Geometry: final body of the model. Coordinates: model frame, mm. Give positions to 0.01 mm unless a question says otherwise; leave off trailing zeros. Order: outer loops, then holes, each group sorted by start corner. A loop starts at its lowest first (then second) coordinate and runs counter-clockwise, first axis right, second up. Notation, with made-up numbers: (-17, -31) -> (8, -31) arc R20 cw to (8, -8) -> close; hole circle Ø2 at (81.5, 83). An arc over 180 degrees is marked (long way). Write item = value, one per line.
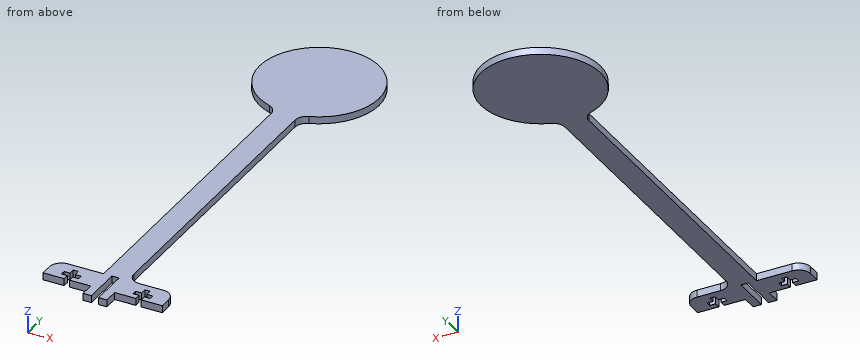
```python
from build123d import *

# Parameters (mm, degrees)
BOSS_EXTRUDE1_DEPTH = 3
FILLET1_R           = 5


with BuildPart() as part:
    # Sketch1 → Boss-Extrude1 (new body)
    with BuildSketch(Plane.XY):
        with BuildLine():
            Line((-5, -25), (-5, -159))
            Line((-5, -159), (-25, -159))
            Line((-25, -159), (-25, -169))
            Line((-25, -169), (-16.1, -169))
            Line((-16.1, -169), (-16.1, -166.5))
            Line((-16.1, -166.5), (-18.6, -166.5))
            Line((-18.6, -166.5), (-18.6, -164.5))
            Line((-18.6, -164.5), (-16.1, -164.5))
            Line((-16.1, -164.5), (-16.1, -162))
            Line((-16.1, -162), (-13.9, -162))
            Line((-13.9, -162), (-13.9, -164.5))
            Line((-13.9, -164.5), (-11.4, -164.5))
            Line((-11.4, -164.5), (-11.4, -166.5))
            Line((-11.4, -166.5), (-13.9, -166.5))
            Line((-13.9, -166.5), (-13.9, -169))
            Line((-13.9, -169), (-5, -169))
            Line((-5, -169), (-5, -175))
            Line((-5, -175), (-1.5, -175))
            Line((-1.5, -175), (-1.5, -159))
            Line((-1.5, -159), (1.5, -159))
            Line((1.5, -159), (1.5, -175))
            Line((1.5, -175), (5, -175))
            Line((5, -175), (5, -169))
            Line((5, -169), (13.9, -169))
            Line((13.9, -169), (13.9, -166.5))
            Line((13.9, -166.5), (11.4, -166.5))
            Line((11.4, -166.5), (11.4, -164.5))
            Line((11.4, -164.5), (13.9, -164.5))
            Line((13.9, -164.5), (13.9, -162))
            Line((13.9, -162), (16.1, -162))
            Line((16.1, -162), (16.1, -164.5))
            Line((16.1, -164.5), (18.6, -164.5))
            Line((18.6, -164.5), (18.6, -166.5))
            Line((18.6, -166.5), (16.1, -166.5))
            Line((16.1, -166.5), (16.1, -169))
            Line((16.1, -169), (25, -169))
            Line((25, -169), (25, -159))
            Line((25, -159), (5, -159))
            Line((5, -159), (5, -25))
            Line((5, -25), (5, -24.494897428))
            ThreePointArc((5, -24.494897428), (0, 25), (-5, -24.494897428))
            Line((-5, -24.494897428), (-5, -25))
        make_face()
    extrude(amount=BOSS_EXTRUDE1_DEPTH)

    # Fillet1
    fillet1_edges = [part.edges().sort_by_distance(p)[0] for p in [
        (5, -24.494897428, 1.5),
        (5, -159, 1.5),
        (25, -159, 1.5),
        (-25, -159, 1.5),
        (-5, -24.494897428, 1.5),
    ]]
    fillet(fillet1_edges, radius=FILLET1_R)


solid = part.part
```
1) Section query B-B (y = -84). Output: boundary loops of the cut face in (x, z), plus the area to 3 significant figures.
Check sheet entries:
outline = (-5, 0) -> (5, 0) -> (5, 3) -> (-5, 3) -> close
area = 30.0 mm²
2) First-contact query: P1, Ø0.9, axis at x = -7.5, z = 2, coming from the -Y side; P2, Ø10, axis at x = 12, y = -109.5, coming from the +Z side; P3, Ø0.9, axis at y = -124.5, z = 1, coming from the -X side; P4, Ø0.7, axis at x = 15.5, z = 1, coming from the -Y side. Flat tips, straight axial feed; report the tip coordinate or a pass-through.
Check sheet entries:
P1 = -169
P2 = through
P3 = -5
P4 = -162
3) Line query: line 1 (X direction, y = -167, z = 1.1); line 2 (Y direction, x = -17, z = 0.6); line 3 (X direction, y = -41.5, z = 1.95). Output: solid intervals per line, ascending. Write a range as from..to.
Check sheet entries:
line_1 = -25..-16.1, -13.9..-1.5, 1.5..13.9, 16.1..25
line_2 = -169..-166.5, -164.5..-159, -18.33..18.33
line_3 = -5..5
4) Section query C-C (y = -19). Output: boundary loops of the cut face in (x, z).
Check sheet entries:
outline = (-16.25, 0) -> (16.25, 0) -> (16.25, 3) -> (-16.25, 3) -> close
5) Section query A-A (x = -22). Output: boundary loops of the cut face in (y, z).
Check sheet entries:
outline = (-169, 0) -> (-159.42, 0) -> (-159.42, 3) -> (-169, 3) -> close; (-11.87, 0) -> (11.87, 0) -> (11.87, 3) -> (-11.87, 3) -> close
